from build123d import *

# Parameters (mm, degrees)
SKETCH001_R       = 4.15
POCKET_DEPTH      = 13.501
POCKET_DEPTH_BACK = -13.501


with BuildPart() as part:
    # Sketch → Revolution (revolve)
    with BuildSketch(Plane.XZ):
        with BuildLine():
            Line((-95, 0), (-95, 12.5))
            Line((-95, 12.5), (-94, 13.5))
            Line((-94, 13.5), (-10, 13.5))
            Line((-10, 13.5), (-4.00316, 12.279929))
            ThreePointArc((0, 7.380306), (-1.128037, 10.543832), (-4.00316, 12.279929))
            Line((0, 7.380306), (0, 0))
            Line((0, 0), (-95, 0))
        make_face()
    revolve(axis=Axis((0, 0, 0), (1, 0, 0)))

    # Sketch001 → Pocket (cut, two sides)
    with BuildSketch(Plane.XY) as pocket_sk:
        with Locations((-85, 0)):
            Circle(SKETCH001_R)
    extrude(amount=-POCKET_DEPTH, mode=Mode.SUBTRACT)
    extrude(pocket_sk.sketch, amount=-POCKET_DEPTH_BACK, mode=Mode.SUBTRACT)


solid = part.part
For this review, take the finished solid that the model builds, in its own axes (mm). Round coordinates to 2 decimals unless told otherwise and drop trailing zeros. Loops run counter-clockwise (first coordinate to the right, second up) from the corner with the lowest first, then second, coordinate; pieces in that order, holes last. Notation, with made-up numbers: (51.25, -25.75) - (89.25, -25.75) arc R27 ccw to (89.25, 0.25) - close; hole circle Ø3 at (31.25, 25.25). An arc over 180 degrees is marked (long way). One line per item, written item: value. Start each with the question number.
Item 1: Clearance check with flat-ended pins moving along their axes: pin 1 Ø2 at (x, z) = (-42.5, -1.5) entering from -Y; pin 2 Ø6.5 at (x, y) = (-85, 0) entering from +Z; pin 3 Ø1.5 at (x, y) = (-70.5, 10.5) entering from -Z; pin 4 Ø4 at (x, y) = (-21, -5.5) entering from -Z. State where each tip first meets the part, or that it passes through.
Item 2: Take a section at C-C (x = -72.5). Give the boundary of the cut face in (y, z), plus the area to 3 significant figures.
Item 3: The part is to be moulded in two halves that separate along Y. For faces 1 (the flat face through (-95, 0, 0)), 2 (the cylindrical face through (-51.41, 5.17, 12.47)), say which applies: +Y half, -Y half, draft (parallel to the pull), parting line (faces both ways), or undercut.
Item 4: For L1, parallel to X at y = 0, z = -3; L2, parallel to Y at x = -85, z = 10; L3, parallel to Y at x = -85, z = -4, list the stretches that pass through material, from the lowest coordinate up.
Item 5: Take a section at A-A (y = 0). Give the boundary of the cut face in (x, z), plus the area to 3 significant figures.
Item 6: Take a section at B-B (x = -85). Give the boundary of the cut face in (y, z).
Answer below:
1. pin 1: stops at y = -13.49
1. pin 2: passes through
1. pin 3: stops at z = -9.34
1. pin 4: stops at z = -13.04
2. outline: circle Ø27 at (0, 0)
2. area: 573 mm2
3. face 1: draft
3. face 2: parting line
4. L1: x = -95 to -89.15, -80.85 to 0
4. L2: y = -9.07 to -4.15, 4.15 to 9.07
4. L3: y = -12.89 to -4.15, 4.15 to 12.89
5. outline: (-95, -12.5) - (-94, -13.5) - (-89.15, -13.5) - (-89.15, 13.5) - (-94, 13.5) - (-95, 12.5) - close; (-80.85, -13.5) - (-10, -13.5) - (-4, -12.28) arc R5 ccw to (0, -7.38) - (0, 7.38) arc R5 ccw to (-4, 12.28) - (-10, 13.5) - (-80.85, 13.5) - close
5. area: 2,310 mm2
6. outline: (-4.15, -12.85) - (-4.15, 12.85) arc R13.5 ccw to start; (4.15, -12.85) arc R13.5 ccw to (4.15, 12.85) - close
